Autodesk Inventor part; units mm, degrees
ref_plane "th1_XY" through (23.8252, 3.9688, 0) normal (0, 0, 1) x (1, 0, 0)
ref_plane "th1_YZ" through (23.8252, 3.9688, 0) normal (1, 0, 0) x (0, 1, 0)
ref_plane "th1_ZX" through (23.8252, 3.9688, 0) normal (0, 1, 0) x (0, 0, 1)
sketch "Sketch_1" plane through (0, 0, 0) normal (0, 0, 1) x (1, 0, 0)
  line L0 (-6.35, 6.35) -> (-6.35, -6.35)
  line L1 (-6.35, -6.35) -> (23.8252, -6.35)
  line L2 (23.8252, -6.35) -> (23.8252, 6.35)
  line L3 (23.8252, 6.35) -> (-6.35, 6.35)
extrude "Extrusion1" add sketch "Sketch_1" along normal mid plane 12.7
sketch "Sketch_2" plane through (0, 0, 0) normal (0, 1, 0) x (-1, 0, 0)
  line L0 (6.35, -3.3338) -> (6.35, 3.3338)
  line L1 (6.35, 3.3338) -> (-11.1252, 3.3338)
  line L2 (-11.1252, 3.3338) -> (-11.1252, -3.3338)
  line L3 (-11.1252, -3.3338) -> (6.35, -3.3338)
extrude "Extrusion2" cut sketch "Sketch_2" along normal mid plane 12.7
sketch "Sketch_3" plane through (0, 0, 0) normal (0, 0, 1) x (1, 0, 0)
  line L0 (23.8252, 0) -> (12.6492, 0)
  line L1 (12.6492, 0) -> (12.6492, 3.396)
  line L2 (12.6492, 3.396) -> (23.2524, 3.396)
  line L3 (23.2524, 3.396) -> (23.8252, 3.9688)
  line L4 (23.8252, 3.9688) -> (23.8252, 0)
  line L5 (23.8252, 0) -> (12.6492, 0)
revolve "Revolution1" cut sketch "Sketch_3" angle 360 about axis through (23.8252, 0, 0) along (1, 0, 0)
thread "Thread1"
sketch "Sketch_4" plane through (0, 0, 0) normal (0, 0, 1) x (1, 0, 0)
  line L0 (12.6492, 0) -> (11.1252, 0)
  line L1 (11.1252, 0) -> (11.1252, 3.396)
  line L2 (11.1252, 3.396) -> (12.6492, 3.396)
  line L3 (12.6492, 3.396) -> (12.6492, 0)
  line L4 (12.6492, 0) -> (11.1252, 0)
revolve "Revolution2" cut sketch "Sketch_4" angle 360 about axis through (12.6492, 0, 0) along (1, 0, 0)
sketch "Sketch_5" plane through (0, 0, 0) normal (1, 0, 0) x (0, 1, 0)
  line L0 (0, -6.35) -> (0, 6.35)
  line L1 (0, 6.35) -> (4.337, 6.35)
  line L2 (4.337, 6.35) -> (3.194, 5.207)
  line L3 (3.194, 5.207) -> (3.194, -5.207)
  line L4 (3.194, -5.207) -> (4.337, -6.35)
  line L5 (4.337, -6.35) -> (0, -6.35)
  line L6 (0, -6.35) -> (0, 6.35)
revolve "Revolution3" cut sketch "Sketch_5" angle 360 about axis through (0, 0, -6.35) along (0, 0, -1)
sketch "Sketch_9" plane through (0, 0, 0) normal (0, 0, 1) x (1, 0, 0)
  line L0 (30.1752, 0) -> (23.8252, 0)
  line L1 (23.8252, 0) -> (23.8252, 6.35)
  arc A0 (23.8252, 6.35) -> (21.2852, 12.7) centre (6.6802, 3.175) ccw
  line L2 (21.2852, 12.7) -> (30.1752, 12.7)
  line L3 (30.1752, 12.7) -> (30.1752, 0)
  line L4 (30.1752, 0) -> (23.8252, 0)
revolve "Revolution4" cut sketch "Sketch_9" angle 360 about axis through (30.1752, 0, 0) along (1, 0, 0)
sketch "Sketch_10" plane through (0, 0, 0) normal (0, 0, 1) x (1, 0, 0)
  line L0 (-6.35, 0) -> (-12.7, 0)
  line L1 (-12.7, 0) -> (-12.7, 12.7)
  line L2 (-12.7, 12.7) -> (-3.81, 12.7)
  arc A0 (-3.81, 12.7) -> (-6.35, 6.35) centre (10.795, 3.175) ccw
  line L3 (-6.35, 6.35) -> (-6.35, 0)
  line L4 (-6.35, 0) -> (-12.7, 0)
revolve "Revolution5" cut sketch "Sketch_10" angle 360 about axis through (-6.35, 0, 0) along (1, 0, 0)
ref_plane "th1_XY" through (23.8252, 3.9688, 0) normal (0, 0, 1) x (1, 0, 0)
ref_plane "th1_YZ" through (23.8252, 3.9688, 0) normal (1, 0, 0) x (0, 1, 0)
ref_plane "th1_ZX" through (23.8252, 3.9688, 0) normal (0, 1, 0) x (0, 0, 1)
ref_plane "th2_XY" through (23.8252, -3.9688, 0) normal (0, 0, 1) x (1, 0, 0)
ref_plane "th2_YZ" through (23.8252, -3.9688, 0) normal (1, 0, 0) x (0, 1, 0)
ref_plane "th2_ZX" through (23.8252, -3.9688, 0) normal (0, 1, 0) x (0, 0, 1)
ref_plane "rod_clevis_body_XY" through (0, 0, 0) normal (0, 0, 1) x (1, 0, 0)
ref_plane "rod_clevis_body_YZ" through (0, 0, 0) normal (1, 0, 0) x (0, 1, 0)
ref_plane "rod_clevis_body_ZX" through (0, 0, 0) normal (0, 1, 0) x (0, 0, 1)
ref_plane "piston_rod_clevis_XY" through (23.8252, 0, 0) normal (1, 0, 0) x (0, 0, -1)
ref_plane "piston_rod_clevis_YZ" through (23.8252, 0, 0) normal (0, 0, -1) x (0, 1, 0)
ref_plane "piston_rod_clevis_ZX" through (23.8252, 0, 0) normal (0, 1, 0) x (1, 0, 0)
ref_plane "dummy_XY" through (0, 0, 0) normal (0, 0, 1) x (1, 0, 0)
ref_plane "dummy_YZ" through (0, 0, 0) normal (1, 0, 0) x (0, 1, 0)
ref_plane "dummy_ZX" through (0, 0, 0) normal (0, 1, 0) x (0, 0, 1)
ref_plane "l11_XY" through (23.8252, 6.35, 0) normal (0, 0, 1) x (1, 0, 0)
ref_plane "l11_YZ" through (23.8252, 6.35, 0) normal (1, 0, 0) x (0, 1, 0)
ref_plane "l11_ZX" through (23.8252, 6.35, 0) normal (0, 1, 0) x (0, 0, 1)
ref_plane "l12_XY" through (0, 6.35, 0) normal (0, 0, 1) x (1, 0, 0)
ref_plane "l12_YZ" through (0, 6.35, 0) normal (1, 0, 0) x (0, 1, 0)
ref_plane "l12_ZX" through (0, 6.35, 0) normal (0, 1, 0) x (0, 0, 1)
ref_plane "l1_XY" through (23.8252, 6.35, 0) normal (0, 0, 1) x (1, 0, 0)
ref_plane "l1_YZ" through (23.8252, 6.35, 0) normal (1, 0, 0) x (0, 1, 0)
ref_plane "l1_ZX" through (23.8252, 6.35, 0) normal (0, 1, 0) x (0, 0, 1)
ref_plane "h1_XY" through (-6.35, 6.35, 0) normal (0, 0, 1) x (1, 0, 0)
ref_plane "h1_YZ" through (-6.35, 6.35, 0) normal (1, 0, 0) x (0, 1, 0)
ref_plane "h1_ZX" through (-6.35, 6.35, 0) normal (0, 1, 0) x (0, 0, 1)
ref_plane "l2_XY" through (-6.35, 6.35, 0) normal (0, 0, 1) x (1, 0, 0)
ref_plane "l2_YZ" through (-6.35, 6.35, 0) normal (1, 0, 0) x (0, 1, 0)
ref_plane "l2_ZX" through (-6.35, 6.35, 0) normal (0, 1, 0) x (0, 0, 1)
ref_plane "h2_XY" through (-6.35, -6.35, 0) normal (0, 0, 1) x (1, 0, 0)
ref_plane "h2_YZ" through (-6.35, -6.35, 0) normal (1, 0, 0) x (0, 1, 0)
ref_plane "h2_ZX" through (-6.35, -6.35, 0) normal (0, 1, 0) x (0, 0, 1)
ref_plane "w11_XY" through (-6.35, 0, -3.3338) normal (0, 1, 0) x (1, 0, 0)
ref_plane "w11_YZ" through (-6.35, 0, -3.3338) normal (1, 0, 0) x (0, 0, -1)
ref_plane "w11_ZX" through (-6.35, 0, -3.3338) normal (0, 0, -1) x (0, 1, 0)
ref_plane "w12_XY" through (-6.35, 0, 3.3338) normal (0, 1, 0) x (1, 0, 0)
ref_plane "w12_YZ" through (-6.35, 0, 3.3338) normal (1, 0, 0) x (0, 0, -1)
ref_plane "w12_ZX" through (-6.35, 0, 3.3338) normal (0, 0, -1) x (0, 1, 0)
ref_plane "l21_XY" through (23.8252, 0, 0) normal (0, 1, 0) x (1, 0, 0)
ref_plane "l21_YZ" through (23.8252, 0, 0) normal (1, 0, 0) x (0, 0, -1)
ref_plane "l21_ZX" through (23.8252, 0, 0) normal (0, 0, -1) x (0, 1, 0)
ref_plane "l22_XY" through (11.1252, 0, 0) normal (0, 1, 0) x (1, 0, 0)
ref_plane "l22_YZ" through (11.1252, 0, 0) normal (1, 0, 0) x (0, 0, -1)
ref_plane "l22_ZX" through (11.1252, 0, 0) normal (0, 0, -1) x (0, 1, 0)
ref_plane "w1_XY" through (23.8252, 0, -6.35) normal (0, 1, 0) x (1, 0, 0)
ref_plane "w1_YZ" through (23.8252, 0, -6.35) normal (1, 0, 0) x (0, 0, -1)
ref_plane "w1_ZX" through (23.8252, 0, -6.35) normal (0, 0, -1) x (0, 1, 0)
ref_plane "w2_XY" through (23.8252, 0, 6.35) normal (0, 1, 0) x (1, 0, 0)
ref_plane "w2_YZ" through (23.8252, 0, 6.35) normal (1, 0, 0) x (0, 0, -1)
ref_plane "w2_ZX" through (23.8252, 0, 6.35) normal (0, 0, -1) x (0, 1, 0)
ref_plane "to_cylinder_XY" through (11.1252, 0, 0) normal (1, 0, 0) x (0, 0, -1)
ref_plane "to_cylinder_YZ" through (11.1252, 0, 0) normal (0, 0, -1) x (0, 1, 0)
ref_plane "to_cylinder_ZX" through (11.1252, 0, 0) normal (0, 1, 0) x (1, 0, 0)
properties part number "D-14059"
Read the model definition and answer for the solid it produces. Units are mm, in the model's axes. A direction names the side the tool comes from. Give positions to 0.01 mm unless a question says otherwise; leave off trailing zeros. Write each loop counter-clockwise with the first axis right and the second up, starting at its lowest first coordinate (ties: lowest second). Pieces come first, ordered by that corner, then holes. Notation, with made-up numbers: (65.25, 10.25) - (69.25, 10.25) arc R20 cw to (69.25, 19.25) - close; hole circle Ø8 at (-22, -3.5). An arc over 180 degrees is marked (long way). Use CSV: the item, a comma, the result in double quotes. Start each with the question number.
(1) Find section C-C (x = 20.5). Give the vertices of the cut face in (y, z).
(2) Determine the mould class of faces 1 (the flat face through (12, -6.35, 0)), 2 (the cylindrical face through (0.959, 3.047, 4.257)), 3 (the flat face through (4, 0, 3.334)), 4 (the flat face through (12, 6.35, 0)) for opening direction Y: +Y half, -Y half, draft (parallel to the pull), parting line (faces both ways), or undercut.
(3) For faces 5 (the flat face through (23.825, -3, 3)), 6 (the flat face through (11.125, -5, 0)), determine the directions among +Z, -Z, +X, -X, +Y, -Y from which every point of the face is accessible in a straight line to the end or side of a thin tool.
(4) Find section A-A (x = 0). Give the vertices of the cut face in (y, z).
(5) Find section B-B (x = 5). Give the vertices of the cut face in (y, z), plus the area to 3 significant figures.
(6) Given P1, Ø1.7, axis at y = -2.5, z = -1.5, coming from the -X side; P2, Ø4, axis at x = 2.5, y = -2, coming from the -Z side, each flat-ended and moving along its own axis, determine where each tip first touches the part or whether it passes through.
(7) Consider line 1 along Y through (x, z) = (20.75, 0); line 2 along Z through (x, y) = (6.5, 5.25). Determine where each line is inside the solid, lowest interval first.
(8) Find section D-D (y = -2). Count the separate pieces of the cut face and the enclosed holes in it, plus the area to 3 significant figures.
Findings below:
1,outline,"(-6.35, -6.35) - (6.35, -6.35) - (6.35, 6.35) - (-6.35, 6.35) - close; hole circle Ø6.79 at (0, 0)"
2,face 1,"-Y half"
2,face 2,"undercut"
2,face 3,"draft"
2,face 4,"+Y half"
3,face 5,"+Z, -Z, +X, +Y, -Y"
3,face 6,"-X, +Y, -Y"
4,outline,"(-6.35, -6.35) - (-4.34, -6.35) - (-3.19, -5.21) - (-3.19, -3.33) - (-6.35, -3.33) - close; (-6.35, 3.33) - (-3.19, 3.33) - (-3.19, 5.21) - (-4.34, 6.35) - (-6.35, 6.35) - close; (3.19, -5.21) - (4.34, -6.35) - (6.35, -6.35) - (6.35, -3.33) - (3.19, -3.33) - close; (3.19, 3.33) - (6.35, 3.33) - (6.35, 6.35) - (4.34, 6.35) - (3.19, 5.21) - close"
5,outline,"(-6.35, -6.35) - (6.35, -6.35) - (6.35, -3.33) - (-6.35, -3.33) - close; (-6.35, 3.33) - (6.35, 3.33) - (6.35, 6.35) - (-6.35, 6.35) - close"
5,area,"76.6 mm2"
6,P1,"x = 11.13"
6,P2,"z = -6.35"
7,line 1,"-6.35 to -3.4, 3.4 to 6.35"
7,line 2,"-6.35 to -3.33, 3.33 to 6.35"
8,separate pieces,"4"
8,enclosed holes,"0"
8,area,"163 mm2"
